Geometry: final body of the model. Coordinates: model frame, mm. A direction names the side the tool comes from. Coordinates: 2 decimals unless noted, no trailing zeros. Order: outer loops, then holes, each group sorted by start corner. A loop starts at its lowest first (then second) coordinate and runs counter-clockwise, first axis right, second up. Notation, with made-up numbers: M 70,21.25 L 122,21.25 A22 ccw 122,49.25 Z; hole C -36.75,45 d4. An arc over 180 degrees is marked long. Use CSV: the item, a comma, the result in double quotes. Start each with the question number.
1. First-contact query: P1, Ø10.5, axis at x = 4.5, y = 3, coming from the +Z side; P2, Ø6.5, axis at y = -37.7, z = 4.05, coming from the +X side; P3, Ø1, axis at x = -25.5, y = 22, coming from the +Z side. Flat tips, straight axial feed; report the tip coordinate or a pass-through.
2. Pull-direction query (Y, two-part tool) for faces 4 (the flat face through (-25, -22, 11.906)), 5 (the flat face through (0, 25.003, 9)), 6 (the flat face through (-18, -25.003, 9)), 7 (the cylindrical face through (-0.089, -35.604, 15.546)); classes: pulls with the +Y half, pulls with the -Y half, needs draft (parallel to the pull), parting line crosses it, or undercut.
3. Material intervals for line 1 (Y direction, x = -25.4, z = 18.75); line 2 (X direction, y = 16, z = 18.5) (3 decimals); line 3 (Y direction, x = 0, z = -0.7), sorted ascending.
4. Section query C-C on z = 2.75. Return the cut outline in (x, y) (3 decimals).
5. Section query A-A on y = 0. Return the cut outline in (x, z) (3 decimals), and give its area (3 significant figures).
6. Section query D-D on x = -10. Return the cut outline in (y, z) (3 decimals).
7. Set-up query: faces 1 (the flat face through (17, -25.003, 9)), 2 (the cylindrical face through (-1.38, -6.2, -1.57)), 3 (the cylindrical face through (-25.744, 20.278, 16.735)). Return all of +Z, -Z, +X, -X, +Y, -Y with unobstructed straight access to the full face (end or side cutting, diameter ignored); none if empty.
8. Section query B-B on x = 2.5. Return the cut outline in (y, z) (3 decimals).
from build123d import *

# Parameters (mm, degrees)
SKETCH1_W           = 57.15
SKETCH1_H           = 50.00625
SKETCH1_W_2         = 44.45
SKETCH1_H_2         = 37.30625
BOSS_EXTRUDE1_DEPTH = 21.43125
SKETCH2_W           = 57.15
SKETCH2_H           = 50.00625
SKETCH2_R           = 6.35
BOSS_EXTRUDE2_DEPTH = 3.175
FILLET1_R           = 1.27
SKETCH6_R           = 1.5875
CUT_EXTRUDE2_DEPTH  = 9.525
SKETCH7_W           = 12.7
SKETCH7_H           = 24.60625
BOSS_EXTRUDE3_DEPTH = 25.4
CUT_EXTRUDE3_REACH  = 66.958
SKETCH8_R           = 2.4892


with BuildPart() as part:
    # Sketch1 → Boss-Extrude1 (new body)
    with BuildSketch(Plane.XY):
        Rectangle(SKETCH1_W, SKETCH1_H)
        Rectangle(SKETCH1_W_2, SKETCH1_H_2, mode=Mode.SUBTRACT)
    extrude(amount=BOSS_EXTRUDE1_DEPTH)

    # Sketch2 → Boss-Extrude2 (add)
    with BuildSketch(Plane.XY):
        Rectangle(SKETCH2_W, SKETCH2_H)
        Circle(SKETCH2_R, mode=Mode.SUBTRACT)
    extrude(amount=-BOSS_EXTRUDE2_DEPTH)

    # Fillet1
    fillet1_edges = [part.edges().sort_by_distance(p)[0] for p in [
        (-22.225, 0, 0),
        (0, -18.653125, 0),
        (22.225, 0, 0),
        (0, 18.653125, 0),
    ]]
    fillet(fillet1_edges, radius=FILLET1_R)

    # Sketch6 → Cut-Extrude2 (cut)
    with BuildSketch(Plane.XY.offset(21.43125)):
        with Locations((-25.4, 21.828125)):
            Circle(SKETCH6_R)
        with Locations((25.4, 21.828125)):
            Circle(SKETCH6_R)
        with Locations((25.4, -21.828125)):
            Circle(SKETCH6_R)
        with Locations((-25.4, -21.828125)):
            Circle(SKETCH6_R)
    extrude(amount=-CUT_EXTRUDE2_DEPTH, mode=Mode.SUBTRACT)

    # Sketch7 → Boss-Extrude3 (add)
    with BuildSketch(Plane.XZ.offset(25.003125)):
        with Locations((0, 9.128125)):
            Rectangle(SKETCH7_W, SKETCH7_H)
    extrude(amount=BOSS_EXTRUDE3_DEPTH)

    # Sketch8 → Cut-Extrude3 (cut, up to next)
    with BuildSketch(Plane.ZY.offset(6.35), mode=Mode.PRIVATE) as cut_extrude3_sk1:
        with Locations((4.048125, -37.703125)):
            Circle(SKETCH8_R)
    cut_extrude3_tool1 = extrude(cut_extrude3_sk1.sketch, amount=-CUT_EXTRUDE3_REACH, mode=Mode.PRIVATE) & part.part
    # Sketch8 → Cut-Extrude3 (cut, up to next)
    with BuildSketch(Plane.ZY.offset(6.35), mode=Mode.PRIVATE) as cut_extrude3_sk2:
        with Locations((14.208125, -37.703125)):
            Circle(SKETCH8_R)
    cut_extrude3_tool2 = extrude(cut_extrude3_sk2.sketch, amount=-CUT_EXTRUDE3_REACH, mode=Mode.PRIVATE) & part.part
    add(cut_extrude3_tool1.solids().sort_by_distance((-6.35, -37.703125, 4.048125))[0], mode=Mode.SUBTRACT)
    add(cut_extrude3_tool2.solids().sort_by_distance((-6.35, -37.703125, 14.208125))[0], mode=Mode.SUBTRACT)


solid = part.part
Results list:
1,P1,"stops at z = 0"
1,P2,"stops at x = 6.35"
1,P3,"stops at z = 11.91"
2,face 4,"undercut"
2,face 5,"pulls with the +Y half"
2,face 6,"pulls with the -Y half"
2,face 7,"undercut"
3,line 1,"y = -25 to -23.42, -20.24 to 20.24, 23.42 to 25"
3,line 2,"x = -28.575 to -22.225, 22.225 to 28.575"
3,line 3,"y = -50.4 to -6.35, 6.35 to 25"
4,outline,"M -28.575,-25.003 L -6.35,-25.003 L -6.35,-35.579 L 6.35,-35.579 L 6.35,-25.003 L 28.575,-25.003 L 28.575,25.003 L -28.575,25.003 Z; M -6.35,-50.403 L 6.35,-50.403 L 6.35,-39.827 L -6.35,-39.827 Z; hole M -22.225,-18.653 L 22.225,-18.653 L 22.225,18.653 L -22.225,18.653 Z"
5,outline,"M -28.575,-3.175 L -6.35,-3.175 L -6.35,0 L -20.955,0 A1.27 cw -22.225,1.27 L -22.225,21.431 L -28.575,21.431 Z; M 6.35,-3.175 L 28.575,-3.175 L 28.575,21.431 L 22.225,21.431 L 22.225,1.27 A1.27 cw 20.955,0 L 6.35,0 Z"
5,area,"414 mm²"
6,outline,"M -25.003,-3.175 L 25.003,-3.175 L 25.003,21.431 L 18.653,21.431 L 18.653,1.27 A1.27 cw 17.383,0 L -17.383,0 A1.27 cw -18.653,1.27 L -18.653,21.431 L -25.003,21.431 Z"
7,face 1,"+Z, -Z, +X, -Y"
7,face 2,"+Z, -Z"
7,face 3,"+Z"
8,outline,"M -50.403,-3.175 L -5.837,-3.175 L -5.837,0 L -17.383,0 A1.27 cw -18.653,1.27 L -18.653,21.431 L -50.403,21.431 Z; M 5.837,-3.175 L 25.003,-3.175 L 25.003,21.431 L 18.653,21.431 L 18.653,1.27 A1.27 cw 17.383,0 L 5.837,0 Z; hole C -37.703,4.048 d4.978; hole C -37.703,14.208 d4.978"
